from build123d import *

# Parameters (mm, degrees)
F0_W     = 108.833484
F0_H     = 82.991742
F1_DEPTH = 25.4
F3_DEPTH = 25.4
F5_DEPTH = 101.6
F6_R     = 15.493018
F7_DEPTH = 82.992742


with BuildPart() as f1:
    # F0 (on Right) → F1 (new body)
    with BuildSketch(Plane.YZ):
        Rectangle(F0_W, F0_H)
    extrude(amount=F1_DEPTH)

    # F2 (on face) → F3 (cut)
    with BuildSketch(Plane.YZ.offset(25.4)):
        Polygon((54.416742, 41.495871), (-23.605434, 41.495871), (54.416742, -41.495871), align=None)
    extrude(amount=-F3_DEPTH, mode=Mode.SUBTRACT)

    # F4 (on face) → F5 (join)
    with BuildSketch(Plane.YZ.offset(25.4)):
        Polygon((-54.416742, 25.108964), (-54.416742, -41.495871), (39.011087, -41.495871), (-23.605434, 25.108964), align=None)
    extrude(amount=F5_DEPTH)

    # F6 (on face) → F7 (cut, through all)
    with BuildSketch(Plane(origin=(0, 0, -41.495871), x_dir=(1, 0, 0), z_dir=(0, 0, -1))):
        with Locations((88.741258, 0)):
            Circle(F6_R)
    extrude(amount=-F7_DEPTH, mode=Mode.SUBTRACT)


solid = f1.part
CAD build for the part. Positions are in the model's coordinates, mm. A direction names the side the tool comes from. Give positions to 0.01 mm unless a question says otherwise; leave off trailing zeros. Write each loop counter-clockwise with the first axis right and the second up, starting at its lowest first coordinate (ties: lowest second). Pieces come first, ordered by that corner, then holes. Notation, with made-up numbers: M 52.5,43.25 L 107.5,43.25 A15 cw 107.5,72.25 Z; hole C 3.25,-29.5 d5. An arc over 180 degrees is marked long. Put each result on its own line as item: value. Start each with the question number.
(1) Flat gauge pins, fed straight in: pin 1 Ø12 at (x, y) = (73.5, -35) entering from +Z; pin 2 Ø10 at (x, y) = (64.5, 4.5) entering from +Z. Where does each tip first touch, or does it go through?
(2) Band-saw the part on A-A, the plane x = 93.5. Write the cut outline in (y, z), and give its area (3 significant figures).
(3) Band-saw the part on D-D, the plane y = -34. Write the cut outline in (x, z), and give its area (3 significant figures).
(4) Band-saw the part on C-C, the plane z = -30.5. Write the cut outline in (x, y).
(5) Probe L1, parallel to X at y = 0, z = -10; L2, parallel to Z at x = 58, y = -26.5; L3, parallel to X at y = 0, z = 4. List the from-to ranges inside material, lowest first.
(6) Which spindle directions (+Z, -Z, +X, -X, +Y, -Y) get a long thin tool onto all of the face, cutting with end or side? Do faces 1 (the face through (25.4, -4, 6)), 2 (the face through (12.88, 14.86, 0.58)), 3 (the face through (75, -39, 25.109)). Say none if no direction does.
(7) Band-saw the part on B-B, the plane y = 3.5. Write the cut outline in (x, z), and give its area (3 significant figures).
(8) Mould opens along Y. For faces 4 (the face through (127, -19, -15)), 5 (the face through (63, -54.417, -9)), 6 (the face through (86.72, -15.36, -19.36)) say: +Y half, -Y half, draft (parallel to the pull), parting line (faces both ways), or undercut.
Response values:
1. pin 1: stops at z = 25.11
1. pin 2: stops at z = 0.53
2. outline: M -54.42,-41.5 L -14.74,-41.5 L -14.74,15.68 L -23.61,25.11 L -54.42,25.11 Z; M 14.74,-41.5 L 39.01,-41.5 L 14.74,-15.68 Z
2. area: 2,910 mm2
3. outline: M 0,-41.5 L 127,-41.5 L 127,25.11 L 25.4,25.11 L 25.4,41.5 L 0,41.5 Z
3. area: 8,880 mm2
4. outline: M 0,-54.42 L 127,-54.42 L 127,28.67 L 25.4,28.67 L 25.4,44.08 L 0,44.08 Z; hole C 88.74,0 d30.99
5. L1: x = 0 to 73.25, 104.23 to 127
5. L2: z = -41.5 to 25.11
5. L3: x = 0 to 25.4
6. face 1: +Z, +X, +Y
6. face 2: +Z, +X, -X, +Y
6. face 3: +Z, +X, +Y, -Y
7. outline: M 0,-41.5 L 73.65,-41.5 L 73.65,-3.72 L 25.4,-3.72 L 25.4,12.66 L 0,12.66 Z; M 103.83,-41.5 L 127,-41.5 L 127,-3.72 L 103.83,-3.72 Z
7. area: 4,070 mm2
8. face 4: draft
8. face 5: -Y half
8. face 6: undercut
